from build123d import *

# Parameters (mm, degrees)
SKETCH1_W           = 32
SKETCH1_H           = 32
BOSS_EXTRUDE1_DEPTH = 8
SKETCH2_W           = 28
SKETCH2_H           = 28
CUT_EXTRUDE1_DEPTH  = 4
SKETCH3_W           = 19
SKETCH3_H           = 19
CUT_EXTRUDE2_DEPTH  = 1.5
SKETCH4_W           = 17
SKETCH4_H           = 17
BOSS_EXTRUDE2_DEPTH = 1.5
SKETCH6_R           = 1.95
BOSS_EXTRUDE3_DEPTH = 6
SKETCH7_R           = 1.5
CUT_EXTRUDE3_DEPTH  = 3


with BuildPart() as part:
    # Sketch1 → Boss-Extrude1 (new body)
    with BuildSketch(Plane(origin=(0, 0, 0), x_dir=(1, 0, 0), z_dir=(0, 1, 0))):
        Rectangle(SKETCH1_W, SKETCH1_H)
    extrude(amount=BOSS_EXTRUDE1_DEPTH)

    # Sketch2 → Cut-Extrude1 (cut)
    with BuildSketch(Plane(origin=(0, 8, 0), x_dir=(1, 0, 0), z_dir=(0, 1, 0))):
        Rectangle(SKETCH2_W, SKETCH2_H)
    extrude(amount=-CUT_EXTRUDE1_DEPTH, mode=Mode.SUBTRACT)

    # Sketch3 → Cut-Extrude2 (cut)
    with BuildSketch(Plane(origin=(0, 4, 0), x_dir=(1, 0, 0), z_dir=(0, 1, 0))):
        Rectangle(SKETCH3_W, SKETCH3_H)
    extrude(amount=-CUT_EXTRUDE2_DEPTH, mode=Mode.SUBTRACT)

    # Sketch4 → Boss-Extrude2 (add)
    with BuildSketch(Plane(origin=(0, 2.5, 0), x_dir=(1, 0, 0), z_dir=(0, 1, 0))):
        Rectangle(SKETCH4_W, SKETCH4_H)
    extrude(amount=BOSS_EXTRUDE2_DEPTH)

    # Sketch6 → Boss-Extrude3 (add)
    with BuildSketch(Plane(origin=(0, 4, 0), x_dir=(1, 0, 0), z_dir=(0, 1, 0))):
        with Locations((-11.75, 11.75)):
            Circle(SKETCH6_R)
        with Locations((11.75, 11.75)):
            Circle(SKETCH6_R)
        with Locations((11.75, -11.75)):
            Circle(SKETCH6_R)
        with Locations((-11.75, -11.75)):
            Circle(SKETCH6_R)
    extrude(amount=BOSS_EXTRUDE3_DEPTH)

    # Sketch7 → Cut-Extrude3 (cut)
    with BuildSketch(Plane(origin=(0, 4, 0), x_dir=(1, 0, 0), z_dir=(0, 1, 0))):
        with Locations((-6, -6)):
            Circle(SKETCH7_R)
        with Locations((-2, -6)):
            Circle(SKETCH7_R)
        with Locations((2, -6)):
            Circle(SKETCH7_R)
        with Locations((6, -6)):
            Circle(SKETCH7_R)
        with Locations((-2, -2)):
            Circle(SKETCH7_R)
        with Locations((2, -2)):
            Circle(SKETCH7_R)
        with Locations((6, -2)):
            Circle(SKETCH7_R)
        with Locations((-2, 2)):
            Circle(SKETCH7_R)
        with Locations((2, 2)):
            Circle(SKETCH7_R)
        with Locations((6, 2)):
            Circle(SKETCH7_R)
        with Locations((-2, 6)):
            Circle(SKETCH7_R)
        with Locations((2, 6)):
            Circle(SKETCH7_R)
        with Locations((6, 6)):
            Circle(SKETCH7_R)
        with Locations((-6, -2)):
            Circle(SKETCH7_R)
        with Locations((-6, 2)):
            Circle(SKETCH7_R)
        with Locations((-6, 6)):
            Circle(SKETCH7_R)
    extrude(amount=-CUT_EXTRUDE3_DEPTH, mode=Mode.SUBTRACT)


solid = part.part
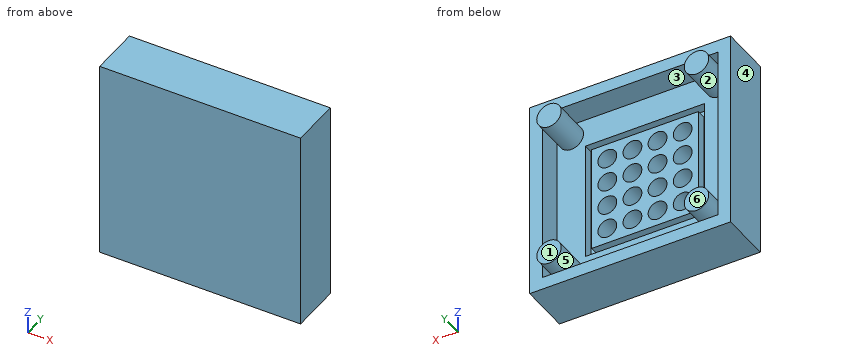
Geometry: final body of the model. Coordinates: model frame, mm. Face numbers are marked on the shaded views. A direction names the side the tool comes from. Give positions to 0.01 mm unless a question says otherwise; leave off trailing zeros. Order: outer loops, then holes, each group sorted by start corner. A loop starts at its lowest first (then second) coordinate and runs counter-clockwise, first axis right, second up. Notation, with made-up numbers: (6.25, -12) -> (45.25, -12) arc R25 cw to (45.25, 11) -> close; hole circle Ø2 at (-16.5, -33). An arc over 180 degrees is marked (long way). Write each question's results on one line, items separated by ' | '.
1) Line query: line 1 along Z through (x, y) = (2, 2.15); line 2 along Z through (x, y) = (5, 1.75). Output: solid intervals per line, ascending.
Geometry says:
line 1: z = -16 to -7.5, -4.5 to -3.5, -0.5 to 0.5, 3.5 to 4.5, 7.5 to 16 | line 2: z = -16 to -7.12, -4.88 to -3.12, -0.88 to 0.88, 3.12 to 4.88, 7.12 to 16
2) First-contact query: pin 1 Ø0.9 at (x, z) = (-6, -6.5) entering from +Y; pin 2 Ø13.5 at (x, z) = (1, 2.5) entering from +Y. Flat tips, straight axial feed; report the tip coordinate or a pass-through.
Geometry says:
pin 1: stops at y = 1 | pin 2: stops at y = 4
3) Draft query along X for the marked faces 1, 2, 3 and 4. Return one class per face: released by +X, released by -X, zero draft, split by the parting line, or undercut.
Geometry says:
face 1: zero draft | face 2: undercut | face 3: undercut | face 4: released by -X
4) Cut plane D-D (z = -8). Output: boundary loops of the cut face in (x, y).
Geometry says:
outline: (-16, 0) -> (16, 0) -> (16, 8) -> (14, 8) -> (14, 4) -> (9.5, 4) -> (9.5, 2.5) -> (8.5, 2.5) -> (8.5, 4) -> (-8.5, 4) -> (-8.5, 2.5) -> (-9.5, 2.5) -> (-9.5, 4) -> (-14, 4) -> (-14, 8) -> (-16, 8) -> close
5) Set-up query: the marked faces 5 and 6. Return all of +Z, -Z, +X, -X, +Y, -Y with unobstructed straight access to the full face (end or side cutting, diameter ignored); none if empty.
Geometry says:
face 5: +Y | face 6: +Z, -Z, +X, -X, +Y
6) Cut plane B-B (z = -11.75). Output: boundary loops of the cut face in (x, y).
Geometry says:
outline: (-16, 0) -> (16, 0) -> (16, 8) -> (14, 8) -> (14, 4) -> (13.7, 4) -> (13.7, 10) -> (9.8, 10) -> (9.8, 4) -> (-9.8, 4) -> (-9.8, 10) -> (-13.7, 10) -> (-13.7, 4) -> (-14, 4) -> (-14, 8) -> (-16, 8) -> close
7) Cut plane A-A (y = 7.25). Output: boundary loops of the cut face in (x, z), and give its area (3 significant figures).
Geometry says:
outline: (-16, -16) -> (16, -16) -> (16, 16) -> (-16, 16) -> close; circle Ø3.9 at (-11.75, -11.75); circle Ø3.9 at (-11.75, 11.75); circle Ø3.9 at (11.75, -11.75); circle Ø3.9 at (11.75, 11.75); hole (-14, -14) -> (14, -14) -> (14, 14) -> (-14, 14) -> close | area: 288 mm²
